Work out the finished part from the listing and answer in its coordinate system (mm). Coordinates: 2 decimals unless noted, no trailing zeros. Write each loop counter-clockwise with the first axis right and the second up, starting at its lowest first coordinate (ties: lowest second). Pieces come first, ordered by that corner, then holes. Notation, with made-up numbers: (43.25, 43) - (99.25, 43) arc R9 cw to (99.25, 60) - close; hole circle Ø10 at (68, 26.25). An arc over 180 degrees is marked (long way). Answer as a JSON object with one key per item and string values. Group by question number.
Autodesk Inventor part; units mm, degrees
ref_plane "YZ Plane" through (0, 0, 0) normal (1, 0, 0) x (0, 1, 0)
ref_plane "XZ Plane" through (0, 0, 0) normal (0, 1, 0) x (-1, 0, 0)
ref_plane "XY Plane" through (0, 0, 0) normal (0, 0, 1) x (1, 0, 0)
sketch "Sketch1" plane through (0, 0, 0) normal (0, 1, 0) x (-1, 0, 0)
  circle A0 centre (-54.4898, 77.8194) radius 1.6
  circle A1 centre (54.4898, 77.8194) radius 1.6
  circle A2 centre (-78.9896, -52.7792) radius 1.6
  circle A3 centre (78.9896, -52.7792) radius 1.6
  line L0 (0, 85) -> (51.2348, 85)
  line L1 (0, 85) -> (-51.2348, 85)
  arc A4 (-53.9313, 84.2105) -> (53.9313, 84.2105) centre (0, 0) ccw
  arc A5 (53.9313, 84.2105) -> (51.2348, 85) centre (51.2348, 80) ccw
  arc A6 (-51.2348, 85) -> (-53.9313, 84.2105) centre (-51.2348, 80) ccw
  point P0 (-54.3117, 78)
  point P1 (54.3117, 78)
  point P2 (52.6783, 85)
  point P3 (-52.6783, 85)
  dimension "d11" = 3.2
  dimension "d12" = 3.2
  dimension "d13" = 3.2
  dimension "d14" = 3.2
  dimension "d20" = 5
extrude "Extrusion1" add sketch "Sketch1" along normal blind 3
properties part number "Top Plate"
Q1. Section C-C on z = 34.5 is taken. Determine the outline of the cut face in (x, y).
Q2. Flat-ended cylindrical pins translate along their axes: pin 1 Ø1 at (y, z) = (1.5, 24.5) entering from +X; pin 2 Ø1.9 at (x, z) = (-54.49, 77.82) entering from +Y. Find the tip coordinate at first contact, or state that the pin passes through.
Q3. Section B-B on x = -85 is taken. Determine the outline of the cut face in (y, z), plus the area to 3 significant figures.
Q4. Section A-A on y = 0.5 is taken. Determine the outline of the cut face in (x, z).
Q5. Consider L1, parallel to X at y = 1, z = -53; L2, parallel to X at y = 0.4, z = 0.5; L3, parallel to Z at x = -53.5, y = 0.4. Determine where each line is inside the solid, lowest interval first. Write a range as from..to.
Numbers:
{
 "1": {"outline": "(-93.86, 0) - (93.86, 0) - (93.86, 3) - (-93.86, 3) - close"},
 "2": {"pin 1": "stops at x = 97.08", "pin 2": "passes through"},
 "3": {"outline": "(0, -52.68) - (3, -52.68) - (3, 52.68) - (0, 52.68) - close", "area": "316 mm²"},
 "4": {"outline": "(-53.93, 84.21) arc R100 ccw (long way) to (53.93, 84.21) arc R5 ccw to (51.23, 85) - (-51.23, 85) arc R5 ccw to start; hole circle Ø3.2 at (-78.99, -52.78); hole circle Ø3.2 at (-54.49, 77.82); hole circle Ø3.2 at (54.49, 77.82); hole circle Ø3.2 at (78.99, -52.78)"},
 "5": {"L1": "x = -84.8..-80.57, -77.4..77.4, 80.57..84.8", "L2": "x = -100..100", "L3": "z = -84.49..76.56, 79.08..84.46"}
}
